Autodesk Inventor part; units mm, degrees
ref_plane "YZ Plane" through (0, 0, 0) normal (1, 0, 0) x (0, 1, 0)
ref_plane "XZ Plane" through (0, 0, 0) normal (0, 1, 0) x (-1, 0, 0)
ref_plane "XY Plane" through (0, 0, 0) normal (0, 0, 1) x (1, 0, 0)
sketch "Skizze1" plane through (0, 0, 0) normal (0, 0, 1) x (1, 0, 0)
  line L0 (3, 11.6) -> (26, 11.6)
  line L1 (26, 11.6) -> (26, -11.6)
  line L2 (26, -11.6) -> (3, -11.6)
  line L3 (0, -8.6) -> (0, 8.6)
  line L4 (-5.9456, 0) -> (31.3243, 0)
  arc A0 (3, 11.6) -> (0, 8.6) centre (3, 8.6) ccw
  arc A1 (0, -8.6) -> (3, -11.6) centre (3, -8.6) ccw
  point P0 (0, 0)
  point P1 (0, 11.6)
  dimension "d0" = 23.2
  dimension "d1" = 26
  dimension "d2" = 3
extrude "Extrusion1" add sketch "Skizze1" along normal blind 3
sketch "Skizze2" plane through (0, 0, 0) normal (0, 0, -1) x (-1, 0, 0)
  line L0 (0, -8.6) -> (0, 8.6)
  arc A0 (0, 8.6) -> (-3, 11.6) centre (-3, 8.6) ccw
  line L1 (-3, 11.6) -> (-26, 11.6)
  line L2 (-26, 11.6) -> (-26, -11.6)
  line L3 (-26, -11.6) -> (-3, -11.6)
  arc A1 (-3, -11.6) -> (0, -8.6) centre (-3, -8.6) ccw
  line L4 (-3, -10.2) -> (-26, -10.2)
  line L5 (-26, -10.2) -> (-26, 10.2)
  line L6 (-26, 10.2) -> (-3, 10.2)
  arc A2 (-1.4, 8.6) -> (-3, 10.2) centre (-3, 8.6) ccw
  line L7 (-1.4, 8.6) -> (-1.4, -8.6)
  arc A3 (-3, -10.2) -> (-1.4, -8.6) centre (-3, -8.6) ccw
  line L8 (0, -8.6) -> (0, 8.6)
  point P0 (0, 0)
  dimension "d8" = 1.4
extrude "Extrusion2" add sketch "Skizze2" along normal blind 1.6 contours A1 L3 L2 L4 A3 L7 A2 L6 L1 A0 L0
sketch "Skizze3" plane through (0, 0, 3) normal (0, 0, 1) x (1, 0, 0)
  line L0 (0, 8.6) -> (0, -8.6)
  arc A0 (0, -8.6) -> (3, -11.6) centre (3, -8.6) ccw
  line L1 (3, -11.6) -> (26, -11.6)
  line L2 (26, -11.6) -> (26, 11.6)
  line L3 (26, 11.6) -> (3, 11.6)
  arc A1 (3, 11.6) -> (0, 8.6) centre (3, 8.6) ccw
  line L4 (0, 8.6) -> (0, -8.6)
  line L5 (0, 3.1) -> (5, 3.1)
  line L6 (5, 3.1) -> (5, -3.1)
  line L7 (5, -3.1) -> (0, -3.1)
  line L8 (0, -3.1) -> (0, 3.1)
  line L9 (-5.6971, 0) -> (31.2828, 0)
  point P0 (0, 0)
  dimension "d9" = 8.5
  dimension "d10" = 5
extrude "Extrusion3" cut sketch "Skizze3" against normal through all contours L5 L6 L9 L0 | L9 L6 L7 L0
sketch "Skizze5" plane through (0, 0, 0) normal (0, 0, -1) x (-1, 0, 0)
  line L0 (-5, -3.1) -> (-5, 3.1)
  line L1 (-31.2, 0) -> (5.2, 0)
  line L2 (-5, 3.1) -> (-5, -3.1)
  line L3 (-5, -3.1) -> (-9.4, -3.1)
  line L4 (-9.4, -3.1) -> (-9.4, 3.1)
  line L5 (-9.4, 3.1) -> (-5, 3.1)
  line L6 (-5, 3.1) -> (-5, -3.1)
  line L7 (-1.4, -8.6) -> (-1.4, -3.1)
  point P0 (0, 0)
  dimension "d23" = 8
extrude "Extrusion4" cut sketch "Skizze5" against normal blind 2
sketch "Skizze4" plane through (0, 0, 0) normal (0, 0, -1) x (-1, 0, 0)
  line L0 (0, -16.24) -> (0, 16.24)
  line L1 (-31.2, 0) -> (5.2, 0)
  line L2 (-1.4, -3.1) -> (-1.4, -8.6)
  point P0 (0, 0)
  point P1 (-5.6, -5)
  point P2 (-5.6, 5)
  dimension "d13" = 10
  dimension "d15" = 4.2
hole "Bohrung1" at (5.6, -5, 0) at (5.6, 5, 0) direction (0, 0, 1) diameter 2 end through all countersink diameter 7 countersink angle 90
fillet "Rundung1" radius 2 2 edges at (5, 3.1, 2.5) (5, -3.1, 2.5)
sketch "Skizze6" plane through (0, 0, -1.6) normal (0, 0, -1) x (-1, 0, 0)
  line L0 (0, -3.1) -> (-1.4, -3.1)
  line L1 (-1.4, -3.1) -> (-1.4, -8.6)
  arc A0 (-3, -10.2) -> (-1.4, -8.6) centre (-3, -8.6) ccw
  line L2 (-3, -10.2) -> (-26, -10.2)
  line L3 (-26, -10.2) -> (-26, -11.6)
  line L4 (-26, -11.6) -> (-3, -11.6)
  arc A1 (-3, -11.6) -> (0, -8.6) centre (-3, -8.6) ccw
  line L5 (0, -8.6) -> (0, -3.1)
  line L6 (-1.4, 3.1) -> (0, 3.1)
  line L7 (0, 3.1) -> (0, 8.6)
  arc A2 (0, 8.6) -> (-3, 11.6) centre (-3, 8.6) ccw
  line L8 (-3, 11.6) -> (-26, 11.6)
  line L9 (-26, 11.6) -> (-26, 10.2)
  line L10 (-26, 10.2) -> (-3, 10.2)
  arc A3 (-1.4, 8.6) -> (-3, 10.2) centre (-3, 8.6) ccw
  line L11 (-1.4, 8.6) -> (-1.4, 3.1)
  line L12 (-3, -11.6) -> (-26, -11.6)
  line L13 (-26, -10.2) -> (-3, -10.2)
  line L14 (-26, -11.6) -> (-21, -11.6)
  line L15 (-21, -11.6) -> (-21, -10.2)
  line L16 (-21, -10.2) -> (-26, -10.2)
  line L17 (-26, -10.2) -> (-26, -11.6)
  point P0 (0, 0)
  dimension "d27" = 5
extrude "Extrusion5" [suppressed]
sketch "Skizze8" plane through (26, -11.6, 3) normal (1, 0, 0) x (0, 0, -1)
  line L0 (0, 23.2) -> (4.6, 23.2)
  line L1 (0, 0) -> (0, 23.2)
  line L2 (0, 0) -> (4.6, 0)
  line L3 (4.6, 1.4) -> (3, 1.4)
  line L4 (3, 21.8) -> (3, 1.4)
  line L5 (3, 21.8) -> (4.6, 21.8)
  line L6 (4.6, 23.2) -> (4.6, 21.8)
  line L7 (6.6, 1.4) -> (5.5, 2.0351)
  line L8 (5.5, 2.0351) -> (4.4, 1.4)
  line L9 (6.6, 1.4) -> (3, 1.4)
  line L10 (5.5, 2.0351) -> (5.5, 1.4) construction
  line L11 (6.6, 1.4) -> (4.4, 1.4)
  line L12 (4.6, 1.4) -> (4.6, 0)
  point P0 (3, 11.6)
  dimension "d30" = 2.2
  dimension "d34" = 30
extrude "Extrusion6" [suppressed]
sketch "Skizze9" plane through (0, 0, -1.6) normal (0, 0, -1) x (-1, 0, 0)
  line L0 (-26, -11.6) -> (-3, -11.6)
  arc A0 (-3, -11.6) -> (0, -8.6) centre (-3, -8.6) ccw
  line L1 (0, -8.6) -> (0, -3.1)
  line L2 (0, -3.1) -> (-1.4, -3.1)
  line L3 (-1.4, -3.1) -> (-1.4, -8.6)
  arc A1 (-3, -10.2) -> (-1.4, -8.6) centre (-3, -8.6) ccw
  line L4 (-3, -10.2) -> (-26, -10.2)
  line L5 (-26, -11.6) -> (-3, -11.6)
  line L6 (-21, -11.6) -> (-20, -11.6)
  line L7 (-20, -11.6) -> (-20, -9.2)
  line L8 (-20, -9.2) -> (-21, -9.2)
  line L9 (-21, -10.6) -> (-21, -11.6)
  line L10 (-20, -9.2) -> (-26, -9.2)
  line L11 (-26, -9.2) -> (-26, -10.6)
  line L12 (-20, -10.2) -> (-20, -9.2)
  line L13 (-21, -10.6) -> (-26, -10.6)
  line L14 (-26, -10.2) -> (-26, -11.6)
  point P0 (0, 0)
  dimension "d40" = 1
  dimension "d41" = 1.4
extrude "Extrusion7" [suppressed]
mirror "Spiegeln1" [suppressed]
chamfer "Fase1" [suppressed]
chamfer "Fase2" distance 0.3 angle 45 6 edges at (14.5, -10.2, -1.6) (1.8686, -9.7314, -1.6) (1.4, -5.85, -1.6) (14.5, 10.2, -1.6) (1.8686, 9.7314, -1.6) (1.4, 5.85, -1.6)
chamfer "Fase3" distance 2 angle 45 2 edges at (0, 3.1, 0.7) (0, -3.1, 0.7)
properties part number "Kondensatorschutz" material "PC/ABS-Kunststoff"
Build history of the part. All positions in model axes, mm. A direction names the side the tool comes from. Coordinates: 2 decimals unless noted, no trailing zeros. Order: outer loops, then holes, each group sorted by start corner. A loop starts at its lowest first (then second) coordinate and runs counter-clockwise, first axis right, second up. Notation, with made-up numbers: (63.5, 46.5) - (111.5, 46.5) arc R18 cw to (111.5, 52.5) - close; hole circle Ø5 at (19, -23.75). An arc over 180 degrees is marked (long way). Put each result on its own line as item: value.
1. Saw through at A-A (z = -0.95). Write the cut outline in (x, y).
Answer sheet:
outline: (0, -8.6) arc R3 ccw to (3, -11.6) - (26, -11.6) - (26, -10.2) - (3, -10.2) arc R1.6 cw to (1.4, -8.6) - (1.4, -3.7) - (0, -5.1) - close; (0, 5.1) - (1.4, 3.7) - (1.4, 8.6) arc R1.6 cw to (3, 10.2) - (26, 10.2) - (26, 11.6) - (3, 11.6) arc R3 ccw to (0, 8.6) - close
2. Pull direction X, two halves, no side cores. Call faces 5 (the face through (1.4, 6, -1)), 6 (the face through (6.031, 6.368, 2.066)), 7 (the face through (6.576, 4.783, 2.754)), 8 (the face through (1, 4.1, 0.7)): pulls with the +X half, pulls with the -X half, needs draft (parallel to the pull), parting line crosses it, or undercut.
Answer sheet:
face 5: pulls with the +X half
face 6: undercut
face 7: undercut
face 8: pulls with the -X half
3. Saw through at D-D (y = -0.5). Write the cut outline in (x, z), and give its area (3 significant figures).
Answer sheet:
outline: (5, 2) - (9.4, 2) - (9.4, 0) - (26, 0) - (26, 3) - (5, 3) - close
area: 54.2 mm^2
4. Saw through at B-B (x = 5.6). Write the cut outline in (y, z), and give its area (4 significant figures).
Answer sheet:
outline: (-11.6, -1.6) - (-10.5, -1.6) - (-10.2, -1.3) - (-10.2, 0) - (-8.5, 0) - (-6, 2.5) - (-6, 3) - (-11.6, 3) - close; (-4, 2.5) - (-3.1, 1.6) - (-3.1, 2) - (3.1, 2) - (3.1, 1.6) - (4, 2.5) - (4, 3) - (-4, 3) - close; (6, 2.5) - (8.5, 0) - (10.2, 0) - (10.2, -1.3) - (10.5, -1.6) - (11.6, -1.6) - (11.6, 3) - (6, 3) - close
area: 39.65 mm^2
5. Saw through at C-C (x = 11.75). Write the cut outline in (y, z).
Answer sheet:
outline: (-11.6, -1.6) - (-10.5, -1.6) - (-10.2, -1.3) - (-10.2, 0) - (10.2, 0) - (10.2, -1.3) - (10.5, -1.6) - (11.6, -1.6) - (11.6, 3) - (-11.6, 3) - close
6. Probe line 1 along Y through (x, z) = (5.6, 2.6); line 2 along Y through (x, z) = (24.75, -0.5); line 3 along Z through (x, y) = (17, 9). List the from-to ranges inside material, lowest first. Write a range as [from, to].
Answer sheet:
line 1: y = [-11.6, -6], [-4, 4], [6, 11.6]
line 2: y = [-11.6, -10.2], [10.2, 11.6]
line 3: z = [0, 3]
7. Drop flat-ended pins along their axis: P1, Ø1, axis at x = 10.5, y = -4, coming from the -Z side; P2, Ø2.5, axis at x = 5.6, y = 5, coming from the -Z side; P3, Ø3, axis at x = 7, y = 1, coming from the -Z side. Give the stop position or say it passes through.
Answer sheet:
P1: stops at z = 0
P2: stops at z = 2.25
P3: stops at z = 2
8. Tool access for faces 1 (the face through (7, 0, 2)), 2 (the face through (1, -4.1, 0.7)), 3 (the face through (14, 11.6, 1)), 4 (the face through (15, 10.2, -1)): list every direction of +Z, -Z, +X, -X, +Y, -Y with a clear straight run to the whole face (end or side of a thin tool).
Answer sheet:
face 1: -Z, -X
face 2: +Z, -Z, -X
face 3: +Z, -Z, +X, -X, +Y
face 4: -Z, +X
